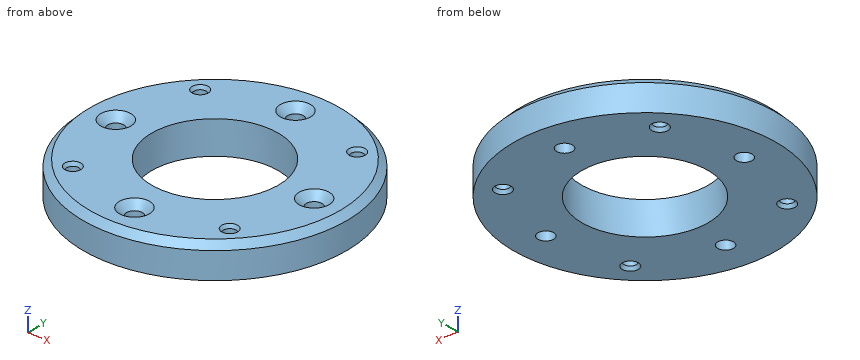
Solid Edge part; units mm, degrees
sketch "Sketch1" plane through (0, 0, 0) normal (0, 0, 1) x (1, 0, 0)
  circle A0 centre (0, 0) radius 40
extrude "Protrusion1" add sketch "Sketch1" along normal blind 10
hole "main_hole" at (0, 0, 10) direction (0, 0, -1) diameter 38.5 end up to next
hole "Hole_2" at (0, 29.6982, 10) direction (0, 0, -1) diameter 4.8 end up to next countersink diameter 9.18 countersink angle 90
hole "Hole_3" at (-23.5, 23.5, 10) direction (0, 0, -1) diameter 3.7 depth 30 tip angle 118 start chamfer 0.6 start chamfer angle 30 end chamfer 0.6 end chamfer angle 30
chamfer "Chamfer_1" distance 2 angle 45 1 edges at (-40, 0, 10)
pattern_circular "Pattern1" count 4 over 360 about axis through (0, 0, 10) along (0, 0, 1) of "Hole_2", "Hole_3"
properties material "Polyethylene, low density"
The model under review builds one solid part; all positions refer to its coordinate system, in mm. Give positions to 0.01 mm unless a question says otherwise; leave off trailing zeros. Write each loop counter-clockwise with the first axis right and the second up, starting at its lowest first coordinate (ties: lowest second). Pieces come first, ordered by that corner, then holes. Notation, with made-up numbers: M 48.25,-10 L 77.25,-10 A12 ccw 77.25,-4 Z; hole C 61.25,34 d6. An arc over 180 degrees is marked long. One line per question, with ' | ' between items. Start each with the question number.
Item 1: For pin 1 (2 mm diameter, centred on y = -17.5, z = 4.5, fed in from -X); pin 2 (1.5 mm diameter, centred on y = -9.5, z = 3.5, fed in from +X); pin 3 (6 mm diameter, centred on x = 0, y = 29.7, fed in from +Z), all flat-tipped, find the tip position at first contact; note any pin that passes through.
Item 2: Wall thickness on line 1 (Y direction, x = 0, z = 2.5); line 2 (Y direction, x = -23.5, z = 7.25); line 3 (Y direction, x = 1.5, z = 7): over which ranges is each line inside the solid? List them lowest first. Write a range as from..to.
Item 3: We need section B-B on z = 4.5. Give the number of separate pieces and of enclosed holes in the cut face, plus the area to 3 significant figures.
Item 4: We need section A-A on y = 0. Write out the cut boundary in (x, z), plus the area to 3 significant figures.
Results found:
1) pin 1: stops at x = -36.44 | pin 2: stops at x = 39.03 | pin 3: stops at z = 8.41
2) line 1: y = -40..-32.1, -27.3..-19.25, 19.25..27.3, 32.1..40 | line 2: y = -32.37..-25.35, -21.65..21.65, 25.35..32.37 | line 3: y = -39.97..-31.57, -27.82..-19.19, 19.19..27.82, 31.57..39.97
3) separate pieces: 1 | enclosed holes: 9 | area: 3,750 mm2
4) outline: M -40,0 L -32.1,0 L -32.1,7.81 L -34.29,10 L -38,10 L -40,8 Z; M -27.3,0 L -19.25,0 L -19.25,10 L -25.11,10 L -27.3,7.81 Z; M 19.25,0 L 27.3,0 L 27.3,7.81 L 25.11,10 L 19.25,10 Z; M 32.1,0 L 40,0 L 40,8 L 38,10 L 34.29,10 L 32.1,7.81 Z | area: 305 mm2
